from build123d import *

# Parameters (mm, degrees)
SKETCH1_R           = 12.5
BOSS_EXTRUDE1_DEPTH = 2
SKETCH2_R           = 1.9
BOSS_EXTRUDE2_DEPTH = 17.5
SKETCH3_R           = 8.5
BOSS_EXTRUDE3_DEPTH = 8.75
SKETCH4_R           = 2
CUT_EXTRUDE1_DEPTH  = 28.834331319
SKETCH5_R           = 5.35
CUT_EXTRUDE2_DEPTH  = 11.5
FILLET1_R           = 0.5
SKETCH6_R           = 2.8
CUT_EXTRUDE3_DEPTH  = 3
FILLET2_R           = 0.25
FILLET3_R           = 10
FILLET4_R           = 10
FILLET5_R           = 10
FILLET6_R           = 10
FILLET7_R           = 10
FILLET8_R           = 10
FILLET9_R           = 1
FILLET10_R          = 0.4


with BuildPart() as part:
    # Sketch1 → Boss-Extrude1 (new body)
    with BuildSketch(Plane(origin=(0, 0, 0), x_dir=(0, 1, 0), z_dir=(0, 0, 1))):
        with Locations(Location((0, 0, 0), (0, 0, 270))):
            Circle(SKETCH1_R)
    boss_extrude1 = extrude(amount=BOSS_EXTRUDE1_DEPTH)

    # Sketch2 → Boss-Extrude2 (add)
    with BuildSketch(Plane.XY.offset(2)):
        with Locations((0, 10.35)):
            Circle(SKETCH2_R)
        with Locations((8.963362929, -5.175)):
            Circle(SKETCH2_R)
        with Locations((-8.963362929, -5.175)):
            Circle(SKETCH2_R)
    extrude(amount=BOSS_EXTRUDE2_DEPTH)

    # Sketch3 → Boss-Extrude3 (add)
    with BuildSketch(Plane.XY.offset(2)):
        Circle(SKETCH3_R)
    boss_extrude3 = extrude(amount=BOSS_EXTRUDE3_DEPTH)

    # Mirror2: Boss-Extrude1, Boss-Extrude3 across plane
    add(boss_extrude1.mirror(Plane.XY.offset(10.75)))
    add(boss_extrude3.mirror(Plane.XY.offset(10.75)))

    # Sketch4 → Cut-Extrude1 (cut, through all)
    with BuildSketch(Plane.XY.offset(21.5)):
        Circle(SKETCH4_R)
    extrude(amount=-CUT_EXTRUDE1_DEPTH, mode=Mode.SUBTRACT)

    # Sketch5 → Cut-Extrude2 (cut)
    with BuildSketch(Plane(origin=(0, 0, 0), x_dir=(1, 0, 0), z_dir=(0, 0, -1))):
        with Locations(Location((0, 0, 0), (0, 0, 180))):
            Circle(SKETCH5_R)
    extrude(amount=-CUT_EXTRUDE2_DEPTH, mode=Mode.SUBTRACT)

    # Fillet1
    fillet1_edges = [part.edges().sort_by_distance(p)[0] for p in [
        (5.35, 0, 0),
    ]]
    fillet(fillet1_edges, radius=FILLET1_R)

    # Sketch6 → Cut-Extrude3 (cut)
    with BuildSketch(Plane.XY.offset(21.5)):
        Circle(SKETCH6_R)
    extrude(amount=-CUT_EXTRUDE3_DEPTH, mode=Mode.SUBTRACT)

    # Fillet2
    fillet2_edges = [part.edges().sort_by_distance(p)[0] for p in [
        (-2.8, 0, 21.5),
    ]]
    fillet(fillet2_edges, radius=FILLET2_R)

    # Fillet3
    fillet3_edges = [part.edges().sort_by_distance(p)[0] for p in [
        (-7.549524157, -3.905724645, 10.75),
    ]]
    fillet(fillet3_edges, radius=FILLET3_R)

    # Fillet4
    fillet4_edges = [part.edges().sort_by_distance(p)[0] for p in [
        (-7.157218842, -4.585217384, 10.75),
    ]]
    fillet(fillet4_edges, radius=FILLET4_R)

    # Fillet5
    fillet5_edges = [part.edges().sort_by_distance(p)[0] for p in [
        (0.392305315, 8.490942029, 10.75),
    ]]
    fillet(fillet5_edges, radius=FILLET5_R)

    # Fillet6
    fillet6_edges = [part.edges().sort_by_distance(p)[0] for p in [
        (-0.392305315, 8.490942029, 10.75),
    ]]
    fillet(fillet6_edges, radius=FILLET6_R)

    # Fillet7
    fillet7_edges = [part.edges().sort_by_distance(p)[0] for p in [
        (7.549524157, -3.905724645, 10.75),
    ]]
    fillet(fillet7_edges, radius=FILLET7_R)

    # Fillet8
    fillet8_edges = [part.edges().sort_by_distance(p)[0] for p in [
        (7.157218842, -4.585217384, 10.75),
    ]]
    fillet(fillet8_edges, radius=FILLET8_R)

    # Fillet9
    # the kernel refuses this fillet: 1 mm, written as the material it takes off along each edge
    with BuildSketch(Plane(origin=(0, 0, 2), x_dir=(1, 0, 0), z_dir=(0, -1, 0))) as fillet9_piece_1_section:
        with BuildLine():
            CenterArc((12.5 - FILLET9_R, -FILLET9_R), FILLET9_R, 0, 90)
            Line((12.5, -FILLET9_R), (12.5, 0))
            Line((12.5, 0), (12.5 - FILLET9_R, 0))
        make_face()
    fillet9_piece_1 = revolve(axis=Axis((0, 0, 2), (0, 0, 1)), mode=Mode.PRIVATE)
    fillet9_piece_1 = fillet9_piece_1 - Plane(origin=(8.963362929, -5.175, 1.726039761), x_dir=(1, 0, 0), z_dir=(0, 0, -1)) * Cylinder(1.9, 51, mode=Mode.PRIVATE)
    fillet9_piece_1 = fillet9_piece_1 - Plane(origin=(-8.963362929, -5.175, 1.726039761), x_dir=(1, 0, 0), z_dir=(0, 0, -1)) * Cylinder(1.9, 51, mode=Mode.PRIVATE)
    fillet9_piece_1 = fillet9_piece_1 - Plane(origin=(0, 10.35, 1.726039761), x_dir=(1, 0, 0), z_dir=(0, 0, -1)) * Cylinder(1.9, 51, mode=Mode.PRIVATE)
    add(fillet9_piece_1, mode=Mode.SUBTRACT)

    # Fillet10
    fillet10_edges = [part.edges().sort_by_distance(p)[0] for p in [
        (5.35, 0, 11.5),
    ]]
    fillet(fillet10_edges, radius=FILLET10_R)


solid = part.part
Can you work these out from the model? Positions are in its coordinate system, mm. A direction names the side the tool comes from. Coordinates: 2 decimals unless noted, no trailing zeros. Use one line per item in the form item = value.
Q1. We'd pull the mould along Z, two halves only. Please class faces 1 (the flat face through (-4.7, 7.5, 19.5)), 2 (the flat face through (-2, -1, 11.5)), 3 (the flat face through (3, -3, 21.5)): +Z half, -Z half, draft (parallel to the pull), parting line (faces both ways), or undercut.
Model answer:
face_1 = undercut
face_2 = -Z half
face_3 = +Z half
Q2. For P1, Ø5, axis at x = 0, y = 0, coming from the -Z side; P2, Ø12, axis at y = -7, z = 9, coming from the -X side; P3, Ø6, axis at y = -6.5, z = 3.5, coming from the -X side, each with a flat end and sliding along its axis, tell me the tip position at first contact or that it passes through.
Model answer:
P1 = 11.5
P2 = -10.86
P3 = -11.63
Q3. I need wall thicknesses on line 1 along Z through (x, y) = (3.5, -8.5); line 2 along Y through (x, z) = (0, 15.25); line 3 along Y through (x, z) = (0, 2.5). Which ranges of each line are inside material? Lowest first, please. Write a range as from..to.
Model answer:
line_1 = 0..2, 19.5..21.5
line_2 = -8.5..-2, 2..12.25
line_3 = -8.5..-5.35, 5.35..12.25
Q4. For faces 4 (the cylindrical face through (0.03, 12.25, 10.46)), 5 (the flat face through (-8, 4, 2)), 6 (the cylindrical face through (-2.8, 0.1, 19.9)), 7 (the flat face through (0, -9, 2)), which set-ups out of +Z, -Z, +X, -X, +Y, -Y let a thin tool reach every point of the face, with its end or its side?
Model answer:
face_4 = +Y
face_5 = -X, +Y
face_6 = +Z
face_7 = -Y
